```python
from build123d import *

# Parameters (mm, degrees)
F0_W     = 25
F0_H     = 20
F1_DEPTH = 10
F3_D     = 6.6
F3_DEPTH = 10
F3_TIP   = 1.9828400428
F5_D     = 5
F5_DEPTH = 30
F5_TIP   = 1.5021515476
F6_R     = 2
F8_D     = 3.3
F8_DEPTH = 6
F8_TIP   = 0.9914200214


with BuildPart() as f1:
    # F0 (on Top) → F1 (new body)
    with BuildSketch(Plane.XY):
        Rectangle(F0_W, F0_H)
    extrude(amount=F1_DEPTH)

    # F3
    with Locations(Plane.XY.offset(10)):
        with Locations((5.5, 0)):
            Hole(F3_D / 2, depth=F3_DEPTH)
            with Locations((0, 0, -(F3_DEPTH + F3_TIP / 2))):  # 118° drill point
                Cone(0, F3_D / 2, F3_TIP, mode=Mode.SUBTRACT)

    # F5
    with Locations(Plane.XZ.offset(10)):
        with Locations((-7, 5), (-1.5, 5)):
            Hole(F5_D / 2, depth=F5_DEPTH)
            with Locations((0, 0, -(F5_DEPTH + F5_TIP / 2))):  # 118° drill point
                Cone(0, F5_D / 2, F5_TIP, mode=Mode.SUBTRACT)

    # F6
    f6_edges = [f1.edges().sort_by_distance(p)[0] for p in [
        (-12.5, -10, 5),
        (-12.5, 10, 5),
        (12.5, -10, 5),
        (12.5, 10, 5),
    ]]
    fillet(f6_edges, radius=F6_R)

    # F8
    with Locations(Plane.XY.offset(10)):
        with Locations((5.5, 7), (5.5, -7)):
            Hole(F8_D / 2, depth=F8_DEPTH)
            with Locations((0, 0, -(F8_DEPTH + F8_TIP / 2))):  # 118° drill point
                Cone(0, F8_D / 2, F8_TIP, mode=Mode.SUBTRACT)


solid = f1.part
```
Geometry: final body of the model. Coordinates: model frame, mm. A direction names the side the tool comes from. Round coordinates to 2 decimals unless told otherwise and drop trailing zeros. Order: outer loops, then holes, each group sorted by start corner. A loop starts at its lowest first (then second) coordinate and runs counter-clockwise, first axis right, second up. Notation, with made-up numbers: (-22, 5) - (-9, 5) arc R33 ccw to (-9, 35) - close; hole circle Ø3 at (-36.5, -37). An arc over 180 degrees is marked (long way). Write item = value, one per line. Start each with the question number.
Q1. Pull-direction query (Y, two-part tool) for faces 1 (the cylindrical face through (2.35, 0.99, 4.93)), 2 (the cylindrical face through (11.9, 9.43, 5.07)), 3 (the cylindrical face through (6.81, 6, 6.96)), 4 (the flat face through (12.5, 0, 5)); classes: +Y half, -Y half, draft (parallel to the pull), parting line (faces both ways), or undercut.
Q2. Cut plane A-A on y = 0. Return the cut outline in (x, z).
Q3. Ray query, line 1 (Y direction, x = 5.5, z = 5.65); line 2 (Z direction, x = -7, y = 3.25); line 3 (X direction, y = -8.5, z = 5.5). Return the intervals inside material, ascending. Write a range as from..to.
Q4. Access query for faces 5 (the cylindrical face through (6.81, -8, 6.96)), 6 (the cylindrical face through (-9.385, 0.14, 5.751)). Directions: +Z, -Z, +X, -X, +Y, -Y. A direction counts if a zero-diameter tool reaches every point of the face in a straight line with its end or side. Return the directions, or none.
Q5. Cut plane C-C on z = 8. Return the cut outline in (x, y), and give its area (3 significant figures).
Q6. Cut plane B-B on z = 5. Return the cut outline in (x, y).
Q7. Pin query (flat end, axial travel): pin 1 (4.5 mm diameter, centred on x = -7, z = 5, fed in from +Y). Return the tip coordinate at first contact, or that it passes through.
Q8. Cut plane D-D on x = -7. Return the cut outline in (y, z), and give its area (3 significant figures).
Outcome:
q1.face_1 = undercut
q1.face_2 = +Y half
q1.face_3 = undercut
q1.face_4 = draft
q2.outline = (-12.5, 0) - (2.2, 0) - (2.2, 10) - (-12.5, 10) - close; (8.8, 0) - (12.5, 0) - (12.5, 10) - (8.8, 10) - close; hole circle Ø5 at (-7, 5); hole circle Ø5 at (-1.5, 5)
q3.line_1 = -10..-8.65, -5.35..-3.3, 3.3..5.35, 8.65..10
q3.line_2 = 0..2.5, 7.5..10
q3.line_3 = -12.44..-9.45, -4.55..-3.95, 0.95..4.81, 6.19..12.44
q4.face_5 = +Z
q4.face_6 = +Y, -Y
q5.outline = (-12.5, -8) arc R2 ccw to (-10.5, -10) - (10.5, -10) arc R2 ccw to (12.5, -8) - (12.5, 8) arc R2 ccw to (10.5, 10) - (-10.5, 10) arc R2 ccw to (-12.5, 8) - close; hole circle Ø6.6 at (5.5, 0); hole circle Ø3.3 at (5.5, -7); hole circle Ø3.3 at (5.5, 7)
q5.area = 445 mm^2
q6.outline = (-12.5, -8) arc R2 ccw to (-10.5, -10) - (-9.5, -10) - (-9.5, 10) - (-10.5, 10) arc R2 ccw to (-12.5, 8) - close; (-4.5, -10) - (-4, -10) - (-4, 10) - (-4.5, 10) - close; (1, -10) - (10.5, -10) arc R2 ccw to (12.5, -8) - (12.5, 8) arc R2 ccw to (10.5, 10) - (1, 10) - close; hole circle Ø6.6 at (5.5, 0); hole circle Ø3.3 at (5.5, -7); hole circle Ø3.3 at (5.5, 7)
q7.pin_1 = through
q8.outline = (-10, 0) - (10, 0) - (10, 2.5) - (-10, 2.5) - close; (-10, 7.5) - (10, 7.5) - (10, 10) - (-10, 10) - close
q8.area = 100 mm^2
